Input: dimensioned drawing with shaded views. Units: mm. Origin: part minimum x, y, z. A direction names the side the tool comes from. Round coordinates to 2 decimals unless told otherwise and drop trailing zeros. Loops run counter-clockwise (first coordinate to the right, second up) from the corner with the lowest first, then second, coordinate; pieces in that order, holes last. Notation, with made-up numbers: M 41.5,-37 L 84.5,-37 A19 ccw 84.5,-21 Z; hole C -2.5,56 d8. An arc over 180 degrees is marked long. Use one line per item in the form item = value. Start each with the question number.
Q1. Section query D-D, the plane y = 16.5. Output: boundary loops of the cut face in (x, z).
Q2. Ray query, line 1 along Y through (x, z) = (8, 3.25); line 2 along X through (y, z) = (26.5, 14); line 3 along X through (y, z) = (98, 12.5). Return the intervals inside material, ascending.
Q3. Access query for the marked faces 1, 2 and 3. Directions: +Z, -Z, +X, -X, +Y, -Y. A direction counts if a zero-diameter tool reaches every point of the face in a straight line with its end or side. Return the directions, or none.
Q4. Section query A-A, the plane z = 14. Output: boundary loops of the cut face in (x, y).
Q5. Section query C-C, the plane y = 66. Output: boundary loops of the cut face in (x, z).
Q6. Section query B-B, the plane x = 14. Output: boundary loops of the cut face in (y, z).
Q7. First-contact query: P1, Ø8, axis at x = 25, y = 92, coming from the -Z side; P2, Ø10, axis at y = 33, z = 13, coming from the +X side; P3, Ø1, axis at x = 11, y = 52.5, coming from the +Z side. Flat tips, straight axial feed; report the tip coordinate or a pass-through.
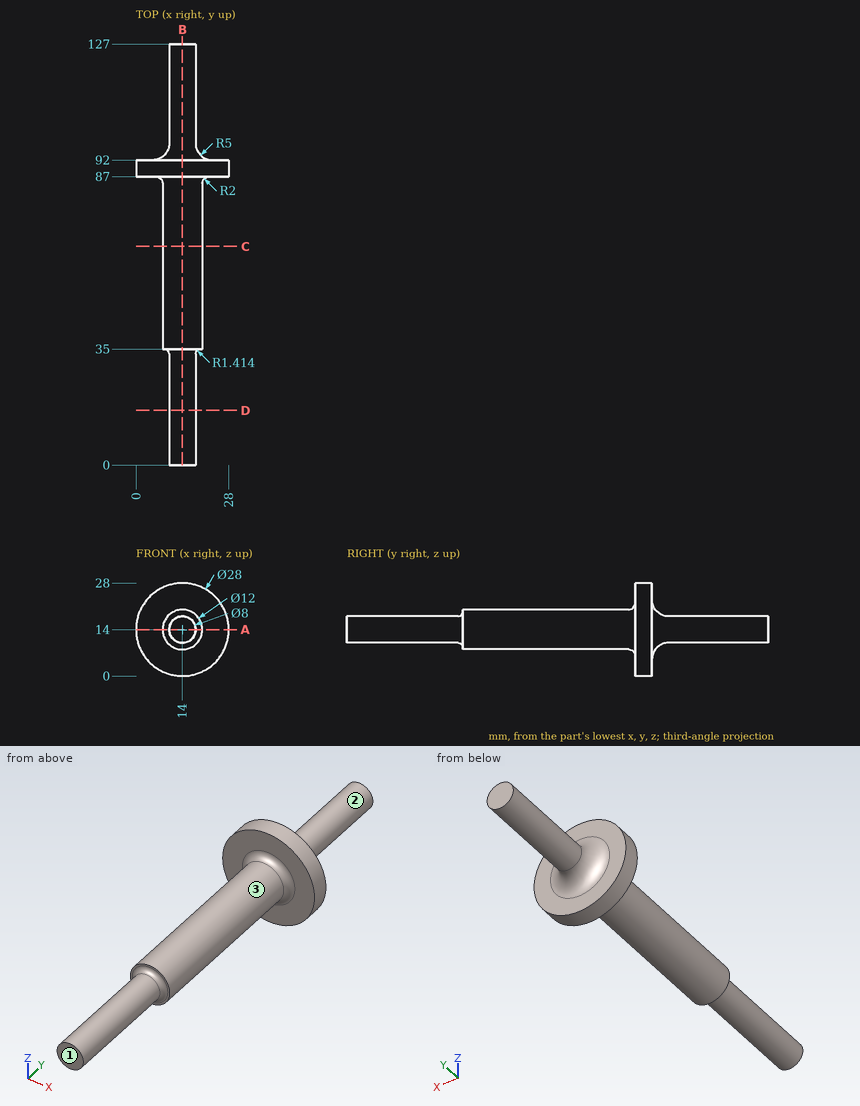
Results found:
q1.outline = C 14,14 d8
q2.line_1 = 87 to 92
q2.line_2 = 10 to 18
q2.line_3 = 10.29 to 17.71
q3.face_1 = +Z, -Z, +X, -X, -Y
q3.face_2 = +Y
q3.face_3 = -Y
q4.outline = M 0,87 L 6,87 A2 cw 8,85 L 8,35 L 8.59,35 A1.41 cw 10,33.59 L 10,0 L 18,0 L 18,33.59 A1.41 cw 19.41,35 L 20,35 L 20,85 A2 cw 22,87 L 28,87 L 28,92 L 23,92 A5 cw 18,97 L 18,127 L 10,127 L 10,97 A5 cw 5,92 L 0,92 Z
q5.outline = C 14,14 d12
q6.outline = M 0,10 L 33.59,10 A1.41 cw 35,8.59 L 35,8 L 85,8 A2 cw 87,6 L 87,0 L 92,0 L 92,5 A5 cw 97,10 L 127,10 L 127,18 L 97,18 A5 cw 92,23 L 92,28 L 87,28 L 87,22 A2 cw 85,20 L 35,20 L 35,19.41 A1.41 cw 33.59,18 L 0,18 Z
q7.P1 = 1.88
q7.P2 = 20
q7.P3 = 19.45
